from build123d import *

# Parameters (mm, degrees)
SKETCH_1_R          = 8.5
EXTRUDE_1_DEPTH     = 2
SKETCH_2_R          = 1.5
CUT_EXTRUDE_1_DEPTH = 10


with BuildPart() as part:
    # 草图1 → 凸台-拉伸1 (new body)
    with BuildSketch(Plane(origin=(0, 0, 0), x_dir=(0, 0, -1), z_dir=(1, 0, 0))):
        with BuildLine():
            ThreePointArc((9.47672316, 7.361502438), (10.778173065, -5.275508068), (0, -12))
            Line((0, -12), (-52.672926825, -12))
            Line((-52.672926825, -12), (-52.672926825, 39.486346501))
            Line((-52.672926825, 39.486346501), (-42.672926825, 39.486346501))
            ThreePointArc((-42.672926825, 39.486346501), (-34.56389856, 50.838013293), (-21.196203665, 46.847848939))
            Line((-21.196203665, 46.847848939), (9.47672316, 7.361502438))
        make_face()
        with Locations((-30.672926825, 39.486346501)):
            Circle(SKETCH_1_R, mode=Mode.SUBTRACT)
        Circle(SKETCH_1_R, mode=Mode.SUBTRACT)
    extrude(amount=EXTRUDE_1_DEPTH)

    # 草图2 → 切除-拉伸1 (cut)
    with BuildSketch(Plane(origin=(2, 0, 0), x_dir=(0, 0, -1), z_dir=(1, 0, 0))):
        with Locations((-47.672926825, 13.74317325)):
            Circle(SKETCH_2_R)
    extrude(amount=-CUT_EXTRUDE_1_DEPTH, mode=Mode.SUBTRACT)


solid = part.part
The listing builds one solid part. Answer for the finished solid, in the listing's coordinates (mm). A direction names the side the tool comes from. Give positions to 0.01 mm unless a question says otherwise; leave off trailing zeros. Write each loop counter-clockwise with the first axis right and the second up, starting at its lowest first coordinate (ties: lowest second). Pieces come first, ordered by that corner, then holes.
1) A tool of negligible diameter and unlimited length cuts with its end or side. For faces 1 (the face through (1, 39.486, 48)), 2 (the face through (0.986, 7.167, -4.57)), from which of +Z, -Z, +X, -X, +Y, -Y can it reach the whole face along a straight path? Write none if from no direction.
2) For a pull along Y with two mould halves and no side action, classify faces 3 (the face through (1, 13, 52.673)), 4 (the face through (0.99, 45.23, 36.94)), 5 (the face through (1, -12, 26)) as pulls with the +Y half, pulls with the -Y half, needs draft (parallel to the pull), parting line crosses it, or undercut.
3) Section A-A (y = 0) is taken. Write down the section's boundary in (x, z), and give its area (3 significant figures).
4) Find the intervals of material crossed by L1, parallel to Z at x = 1.5, y = -5.5; L2, parallel to Y at x = 1.8, z = 36.5; L3, parallel to Z at x = 1.5, y = -2, in increasing order.
5) Section D-D (y = 27.5) is taken. Write down the section's boundary in (x, z), and give its area (3 significant figures).
6) Section B-B (z = 35.5) is taken. Write down the section's boundary in (x, y).
7) Given P1, Ø10, axis at y = 39.49, z = 30.67, coming from the -X side; P2, Ø1, axis at x = 1, z = 48.5, coming from the +Y side; P3, Ø1, axis at x = 0.5, y = 1, coming from the -Z side, each flat-ended and moving along its own axis, determine where each tip first touches the part or whether it passes through.
8) Section C-C (x = 1.3) is taken. Write down the section's boundary in (y, z).
Response:
1. face 1: +Z, +X, -X, +Y
1. face 2: +X, -X
2. face 3: needs draft
2. face 4: undercut
2. face 5: pulls with the -Y half
3. outline: (0, -12) - (2, -12) - (2, -8.5) - (0, -8.5) - close; (0, 8.5) - (2, 8.5) - (2, 52.67) - (0, 52.67) - close
3. area: 95.3 mm2
4. L1: z = -10.67 to -6.48, 6.48 to 52.67
4. L2: y = -12 to 33.3, 45.67 to 49.98
4. L3: z = -11.83 to -8.26, 8.26 to 52.67
5. outline: (0, 6.17) - (2, 6.17) - (2, 52.67) - (0, 52.67) - close
5. area: 93.0 mm2
6. outline: (0, -12) - (2, -12) - (2, 32.49) - (0, 32.49) - close; (0, 46.48) - (2, 46.48) - (2, 50.47) - (0, 50.47) - close
7. P1: passes through
7. P2: stops at y = 39.49
7. P3: stops at z = -11.99
8. outline: (-12, 0) arc R12 ccw to (7.36, -9.48) - (46.85, 21.2) arc R12 ccw to (39.49, 42.67) - (39.49, 52.67) - (-12, 52.67) - close; hole circle Ø17 at (0, 0); hole circle Ø3 at (13.74, 47.67); hole circle Ø17 at (39.49, 30.67)
